```python
from build123d import *

# Parameters (mm, degrees)
F0_W         = 75
F0_H         = 40
F1_DEPTH     = 25
F2_R         = 4
F3_DEPTH     = 25
F4_R         = 5
F5_T1_DEPTH  = 27.5
F5_T3_DEPTH  = 65
F5_T5_DEPTH  = 47.5
F5_T7_DEPTH  = 100
F5_S11_W     = 5.1
F5_S11_H     = 5.1
F5_T12_DEPTH = 5.1
F5_S17_W     = 5.1
F5_S17_H     = 5.1
F5_T18_DEPTH = 5.1


# Not quite as in the source:
# - a fillet or chamfer that OpenCascade refuses, or shapes differently, is made with other operations: its cross-section is extruded or revolved along the edge and cut away or added


with BuildPart() as f1:
    # F0 (on Front) → F1 (new body)
    with BuildSketch(Plane.XZ):
        Rectangle(F0_W, F0_H)
    extrude(amount=F1_DEPTH)

    # F2 (on face) → F3 (cut)
    with BuildSketch(Plane.XZ.offset(25)):
        Circle(F2_R)
    extrude(amount=-F3_DEPTH, mode=Mode.SUBTRACT)

    # F4
    f4_edges = [f1.edges().sort_by_distance(p)[0] for p in [
        (0, -25, 20),
        (-37.5, -25, 0),
        (0, -25, -20),
        (37.5, -25, 0),
    ]]
    fillet(f4_edges, radius=F4_R)

    # F5: fillet of radius 5 on 8 edges, made by hand

    # F5_s2 → F5_t1 (cut)
    with BuildSketch(Plane.XZ.offset(5)):
        with BuildLine():
            ThreePointArc((-32.5, -20), (-36.0355339059, -18.5355339059), (-37.5, -15))
            Line((-37.5, -15), (-37.5, -20))
            Line((-37.5, -20), (-32.5, -20))
        make_face()
        with BuildLine():
            ThreePointArc((37.5, -15), (36.0355339059, -18.5355339059), (32.5, -20))
            Line((32.5, -20), (37.5, -20))
            Line((37.5, -20), (37.5, -15))
        make_face()
    extrude(amount=F5_T1_DEPTH, mode=Mode.SUBTRACT)

    # F5_s4 → F5_t3 (cut)
    with BuildSketch(Plane.YZ.offset(-32.5)):
        with BuildLine():
            ThreePointArc((-5, -20), (-1.4644660941, -18.5355339059), (0, -15))
            Line((0, -15), (0, -20))
            Line((0, -20), (-5, -20))
        make_face()
    extrude(amount=F5_T3_DEPTH, mode=Mode.SUBTRACT)

    # F5_s6 → F5_t5 (cut)
    with BuildSketch(Plane.XY.offset(-15)):
        with BuildLine():
            ThreePointArc((37.5, -5), (36.0355339059, -1.4644660941), (32.5, 0))
            Line((32.5, 0), (37.5, 0))
            Line((37.5, 0), (37.5, -5))
        make_face()
        with BuildLine():
            ThreePointArc((-32.5, 0), (-36.0355339059, -1.4644660941), (-37.5, -5))
            Line((-37.5, -5), (-37.5, 0))
            Line((-37.5, 0), (-32.5, 0))
        make_face()
    extrude(amount=F5_T5_DEPTH, mode=Mode.SUBTRACT)

    # F5_s8 → F5_t7 (cut)
    with BuildSketch(Plane.YZ.offset(-50)):
        with BuildLine():
            ThreePointArc((0, 15), (-1.4644660941, 18.5355339059), (-5, 20))
            Line((-5, 20), (0, 20))
            Line((0, 20), (0, 15))
        make_face()
    extrude(amount=F5_T7_DEPTH, mode=Mode.SUBTRACT)


with BuildPart() as f5_tool10:
    # F5_s11 → F5_t12 (new body)
    with BuildSketch(Plane.XY.offset(-15)):
        with Locations((-35.05, -2.45)):
            Rectangle(F5_S11_W, F5_S11_H)
    extrude(amount=-F5_T12_DEPTH)

    # F5_s13 → F5_t14 (revolve, cut)
    with BuildSketch(Plane(origin=(-32.5, -5, -15), x_dir=(0.7071067812, -0.7071067812, 0), z_dir=(0.7071067812, 0.7071067812, 0))):
        with BuildLine():
            ThreePointArc((0, -5), (5, 0), (0, 5))
            Line((0, 5), (0, -5))
        make_face()
    revolve(axis=Axis((-32.5, -5, -15), (0, 0, -1)), mode=Mode.SUBTRACT)


with BuildPart() as f1_1:
    add(f1.part)

    # F5_t9: cut F5_tool10
    add(f5_tool10.part, mode=Mode.SUBTRACT)


with BuildPart() as f5_tool16:
    # F5_s17 → F5_t18 (new body)
    with BuildSketch(Plane.YZ.offset(32.5)):
        with Locations((-2.45, -17.55)):
            Rectangle(F5_S17_W, F5_S17_H)
    extrude(amount=F5_T18_DEPTH)

    # F5_s19 → F5_t20 (revolve, cut)
    with BuildSketch(Plane(origin=(32.5, -5, -15), x_dir=(0, -0.7071067812, 0.7071067812), z_dir=(0, 0.7071067812, 0.7071067812))):
        with BuildLine():
            ThreePointArc((0, -5), (5, 0), (0, 5))
            Line((0, 5), (0, -5))
        make_face()
    revolve(axis=Axis((32.5, -5, -15), (1, 0, 0)), mode=Mode.SUBTRACT)


with BuildPart() as f1_2:
    add(f1_1.part)

    # F5_t15: cut F5_tool16
    add(f5_tool16.part, mode=Mode.SUBTRACT)

    # F5_s21 → F5_t22 (revolve, cut)
    with BuildSketch(Plane.XY):
        with BuildLine():
            ThreePointArc((9, -25), (5.4644660941, -23.5355339059), (4, -20))
            Line((4, -20), (4, -25))
            Line((4, -25), (9, -25))
        make_face()
    revolve(axis=Axis((0, -25, 0), (0, -1, 0)), mode=Mode.SUBTRACT)


solid = f1_2.part
```
The model under review builds one solid part; all positions refer to its coordinate system, in mm. Give positions to 0.01 mm unless a question says otherwise; leave off trailing zeros. Write each loop counter-clockwise with the first axis right and the second up, starting at its lowest first coordinate (ties: lowest second). Pieces come first, ordered by that corner, then holes. Notation, with made-up numbers: (-9.75, 60.25) -> (-1.75, 60.25) arc R35 cw to (-1.75, 98.25) -> close; hole circle Ø10 at (35.5, 80.5). An arc over 180 degrees is marked (long way). Put each result on its own line as item: value.
(1) We need section A-A, the plane x = 0. Give the boundary of the cut face in (y, z).
Results are:
outline: (-25, -15) arc R5 ccw to (-20, -20) -> (-5, -20) arc R5 ccw to (0, -15) -> (0, -4) -> (-20, -4) arc R5 ccw to (-25, -9) -> close; (-25, 9) arc R5 ccw to (-20, 4) -> (0, 4) -> (0, 15) arc R5 ccw to (-5, 20) -> (-20, 20) arc R5 ccw to (-25, 15) -> close
(2) We need section B-B, the plane y = -6. Give the boundary of the cut face in (x, z), and give its area (3 significant figures).
Results are:
outline: (-37.5, -15) arc R5 ccw to (-32.5, -20) -> (32.5, -20) arc R5 ccw to (37.5, -15) -> (37.5, 20) -> (-37.5, 20) -> close; hole circle Ø8 at (0, 0)
area: 2,940 mm²
(3) We need section C-C, the plane z = 0. Give the boundary of the cut face in (x, y), and give its area (3 significant figures).
Results are:
outline: (-37.5, -20) arc R5 ccw to (-32.5, -25) -> (-9, -25) arc R5 ccw to (-4, -20) -> (-4, 0) -> (-32.5, 0) arc R5 ccw to (-37.5, -5) -> close; (4, -20) arc R5 ccw to (9, -25) -> (32.5, -25) arc R5 ccw to (37.5, -20) -> (37.5, -5) arc R5 ccw to (32.5, 0) -> (4, 0) -> close
area: 1,640 mm²
(4) We need section D-D, the plane x = -31. Give the boundary of the cut face in (y, z), and give its area (3 significant figures).
Results are:
outline: (-25, -15) arc R5 ccw to (-20, -20) -> (-5, -20) arc R5 ccw to (0, -15) -> (0, 15) arc R5 ccw to (-5, 20) -> (-20, 20) arc R5 ccw to (-25, 15) -> close
area: 979 mm²
(5) To check wall thickness, follow probe 1 along Z at (x, y) = (0, -7.25); probe 2 along Z at (x, y) = (1, -11); probe 3 along X at (y, z) = (-2.5, 14.5). State the ranges of each line that lie inside material, in increasing order. Write a range as from..to.
Results are:
probe 1: -20..-4, 4..20
probe 2: -20..-3.87, 3.87..20
probe 3: -36.83..36.83
